For this review, take the finished solid that the model builds, in its own axes (mm). Face numbers are marked on the shaded views. Give positions to 0.01 mm unless a question says otherwise; leave off trailing zeros. Write each loop counter-clockwise with the first axis right and the second up, starting at its lowest first coordinate (ties: lowest second). Pieces come first, ordered by that corner, then holes.
Q1. We need section A-A (y = 0). Write out the cut boundary in (x, z).
Q2. Insertion check: P1, Ø2.5, axis at x = 0.5, z = 10, coming from the -Y side; P2, Ø0.9, axis at y = 8, z = 10.5, coming from the +X side; P3, Ø0.9, axis at x = -8, z = 11, coming from the +Y side; P4, Ø3, axis at x = 0, y = 0, coming from the -Z side. Each pin has a flat end and moves straight along its axis. Give the tip position at first contact, or say it passes through.
Q3. We need section C-C (x = 21.5). Write out the cut boundary in (y, z), then the cut area to 3 significant figures.
Q4. We need section D-D (z = 4.5). Write out the cut boundary in (x, y), then the cut area to 3 significant figures.
Q5. Mouldability with a two-part tool opening along Z and no side actions: class the marked faces 1 and 2 as released by +Z, released by -Z, zero draft, split by the parting line, or undercut.
Q6. For line 1 (Y direction, x = 0, z = 4.5); line 2 (Z direction, x = -25.5, y = -12.5); line 3 (Z direction, x = -10, y = 5.5), list the stretches that pass through material, from the lowest coordinate up.
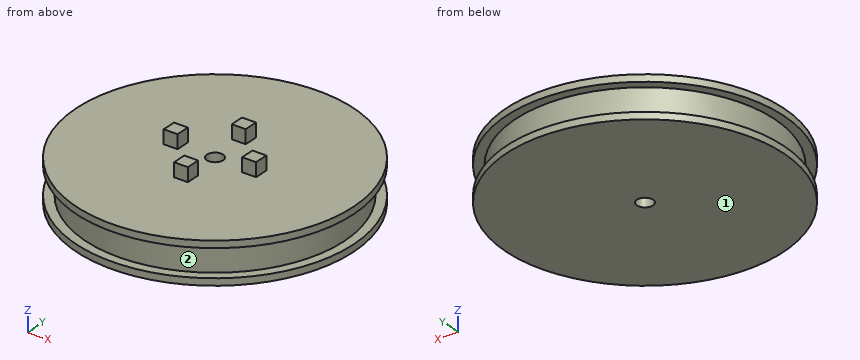
```python
from build123d import *

# Parameters (mm, degrees)
F3_DEPTH = 3
F4_DEPTH = 3


with BuildPart() as f1:
    # F0 (on Front) → F1 (revolve)
    with BuildSketch(Plane.XZ):
        Polygon((1.75, 9), (1.75, 0), (27.950706, 0), (30, 0), (30, 1.5), (28, 1.5), (28, 7.5), (30, 7.5), (30, 9), align=None)
    revolve(axis=Axis((0, 0, 5), (0, 0, 1)))

    # F2 (on face) → F3 (join)
    with BuildSketch(Plane.XY.offset(9)):
        Polygon((-1.5, 7), (1.5, 7), (1.5, 10), (0, 10), (-1.5, 10), align=None)
        Polygon((1.5, -7), (-1.5, -7), (-1.5, -10), (0, -10), (1.5, -10), align=None)
        Polygon((-7, -1.5), (-7, 1.5), (-10, 1.5), (-10, 0), (-10, -1.5), align=None)
        Polygon((10, -1.5), (10, 0), (10, 1.5), (7, 1.5), (7, -1.5), align=None)
    extrude(amount=F3_DEPTH)

    # F2 (on face) → F4 (join)
    with BuildSketch(Plane.XY.offset(9)):
        Polygon((-1.5, 7), (1.5, 7), (1.5, 10), (0, 10), (-1.5, 10), align=None)
        Polygon((-7, -1.5), (-7, 1.5), (-10, 1.5), (-10, 0), (-10, -1.5), align=None)
        Polygon((1.5, -7), (-1.5, -7), (-1.5, -10), (0, -10), (1.5, -10), align=None)
        Polygon((10, -1.5), (10, 0), (10, 1.5), (7, 1.5), (7, -1.5), align=None)
    extrude(amount=F4_DEPTH)


solid = f1.part
```
Computed:
1. outline: (-30, 0) - (-1.75, 0) - (-1.75, 9) - (-7, 9) - (-7, 12) - (-10, 12) - (-10, 9) - (-30, 9) - (-30, 7.5) - (-28, 7.5) - (-28, 1.5) - (-30, 1.5) - close; (1.75, 0) - (30, 0) - (30, 1.5) - (28, 1.5) - (28, 7.5) - (30, 7.5) - (30, 9) - (10, 9) - (10, 12) - (7, 12) - (7, 9) - (1.75, 9) - close
2. P1: stops at y = -30
2. P2: stops at x = 1.5
2. P3: stops at y = 1.5
2. P4: passes through
3. outline: (-20.92, 0) - (20.92, 0) - (20.92, 1.5) - (17.94, 1.5) - (17.94, 7.5) - (20.92, 7.5) - (20.92, 9) - (-20.92, 9) - (-20.92, 7.5) - (-17.94, 7.5) - (-17.94, 1.5) - (-20.92, 1.5) - close
3. area: 341 mm2
4. outline: circle Ø56 at (0, 0); hole circle Ø3.5 at (0, 0)
4. area: 2,450 mm2
5. face 1: released by -Z
5. face 2: undercut
6. line 1: y = -28 to -1.75, 1.75 to 28
6. line 2: z = 0 to 1.5, 7.5 to 9
6. line 3: z = 0 to 9
